CAD build for the part. Positions are in the model's coordinates, mm. Face numbers are marked on the shaded views. A direction names the side the tool comes from. Round coordinates to 2 decimals unless told otherwise and drop trailing zeros. Order: outer loops, then holes, each group sorted by start corner. A loop starts at its lowest first (then second) coordinate and runs counter-clockwise, first axis right, second up. Notation, with made-up numbers: (78.25, 19.5) - (108.25, 19.5) arc R8 cw to (108.25, 24.5) - close; hole circle Ø1 at (40, 73). An arc over 180 degrees is marked (long way). Write item = value, one per line.
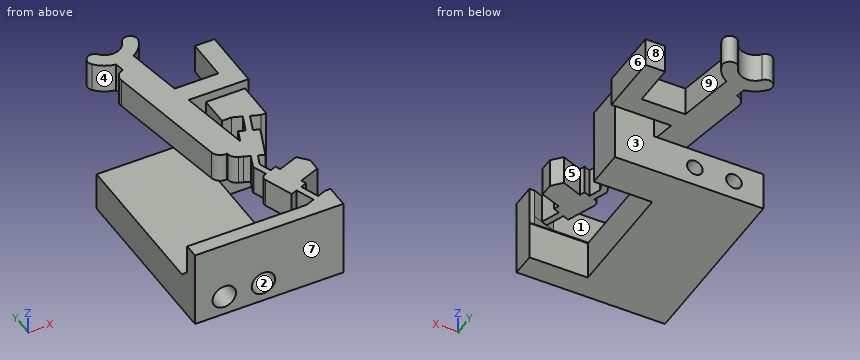
from build123d import *

# Parameters (mm, degrees)
BOSS_SWITCH_BODY_DEPTH            = 3
SKETCH1_W                         = 2.994375291
SKETCH1_H                         = 2.409101515
SKETCH1_W_2                       = 3.994375291
SKETCH1_H_2                       = 3.957767538
BOSS_FLANGE_WIDTH_DEPTH           = 5
BOSS_FLANGE_HEIGHT_REACH          = 36.354
SKETCH2_W                         = 4
SKETCH2_H                         = 3.957767538
SKETCH2_W_2                       = 8
SKETCH2_H_2                       = 1.451333978
SKETCH17_W                        = 15.1675
SKETCH17_H                        = 4
BOSS_FLANGE_SUPPORT_DEPTH         = 13.053634428
CUT_WALL_GAP_DEPTH                = 1
TAP_DRILL_FOR_M2X0_4_TAP1_D       = 1.6
M2_CLEARANCE_HOLE2_D              = 2.4
M2_CLEARANCE_HOLE2_DEPTH          = 13.462735941
CHAMFER_FLANGE_SUPPORT_3_SIZE     = 1
FILLET1_R                         = 1
FILLET2_R                         = 0.5
SKETCH28_W                        = 5.9675
SKETCH28_H                        = 12.095866891
CUT_PRINT_SUPPORT_CLEARANCE_DEPTH = 33.624103931


with BuildPart() as part:
    # Sketch-SwitchBossUp → Boss-Switch Body (new body)
    with BuildSketch(Plane.XY):
        with BuildLine():
            Line((-5.697895702, 26.949658376), (-5.524247524, 25.964850623))
            ThreePointArc((-5.524247524, 25.964850623), (-6.169751391, 25.553619307), (-6.3354071, 24.806394693))
            Line((-6.3354071, 24.806394693), (-4.07798079, 12.003893904))
            ThreePointArc((-4.07798079, 12.003893904), (-3.666749473, 11.358390037), (-2.919524859, 11.192734328))
            Line((-2.919524859, 11.192734328), (-2.795819507, 10.49116641))
            Line((-2.795819507, 10.49116641), (-1.8481327, 10.123820116))
            Line((-1.8481327, 10.123820116), (-1.21876104, 9.87986046))
            Line((-1.21876104, 9.87986046), (-1.735258621, 8.547390389))
            ThreePointArc((-1.735258621, 8.547390389), (-1.752158006, 8.457034961), (-1.735258621, 8.366679532))
            Line((-1.735258621, 8.366679532), (-1.21876104, 7.034209461))
            Line((-1.21876104, 7.034209461), (-1.8481327, 6.790249805))
            Line((-1.8481327, 6.790249805), (-0.547014535, 3.433600952))
            Line((-0.547014535, 3.433600952), (0.082357125, 3.677560608))
            Line((0.082357125, 3.677560608), (0.805200549, 1.81275569))
            Line((0.805200549, 1.81275569), (-0.12720191, 1.451333978))
            Line((-0.12720191, 1.451333978), (-0.12720191, 0))
            Line((-0.12720191, 0), (2.867173381, 0))
            Line((2.867173381, 0), (2.867173381, 2.409101515))
            Line((2.867173381, 2.409101515), (2.343664607, 2.409101515))
            Line((2.343664607, 2.409101515), (1.411262148, 2.047679803))
            Line((1.411262148, 2.047679803), (0.688418723, 3.912484721))
            Line((0.688418723, 3.912484721), (1.317790383, 4.156444377))
            Line((1.317790383, 4.156444377), (1.117265944, 4.673761056))
            Line((1.117265944, 4.673761056), (3.17940291, 5.473095148))
            Line((3.17940291, 5.473095148), (3.17940291, 6.808547192))
            Line((3.17940291, 6.808547192), (2.279218661, 7.795066081))
            Line((2.279218661, 7.795066081), (0.217196658, 6.995776551))
            Line((0.217196658, 6.995776551), (0.016672219, 7.51309323))
            Line((0.016672219, 7.51309323), (-0.612699441, 7.269133574))
            Line((-0.612699441, 7.269133574), (-1.038134762, 8.366679532))
            ThreePointArc((-1.038134762, 8.366679532), (-1.055034148, 8.457034961), (-1.038134762, 8.547390389))
            Line((-1.038134762, 8.547390389), (-0.612699441, 9.644936347))
            Line((-0.612699441, 9.644936347), (0.016672219, 9.400976691))
            Line((0.016672219, 9.400976691), (1.317790383, 12.757625544))
            Line((1.317790383, 12.757625544), (0.688418723, 13.0015852))
            Line((0.688418723, 13.0015852), (1.411262148, 14.866390118))
            Line((1.411262148, 14.866390118), (2.343664607, 14.504968406))
            Line((2.343664607, 14.504968406), (2.867173381, 14.504968406))
            Line((2.867173381, 14.504968406), (2.867173381, 18.462735944))
            Line((2.867173381, 18.462735944), (-0.111637615, 18.462735944))
            Line((-0.111637615, 18.462735944), (-1.12720191, 18.462735944))
            Line((-1.12720191, 18.462735944), (-1.12720191, 15.462735944))
            Line((-1.12720191, 15.462735944), (-0.12720191, 15.462735944))
            Line((-0.12720191, 15.462735944), (0.805200549, 15.101314231))
            Line((0.805200549, 15.101314231), (0.082357125, 13.236509313))
            Line((0.082357125, 13.236509313), (-0.547014535, 13.480468969))
            Line((-0.547014535, 13.480468969), (-1.059112089, 12.159350171))
            Line((-1.059112089, 12.159350171), (-2.346896051, 19.462735944))
            Line((-2.346896051, 19.462735944), (3.767173381, 19.462735944))
            Line((3.767173381, 19.462735944), (3.767173381, 25.857619356))
            Line((3.767173381, 25.857619356), (1.767173381, 25.857619356))
            Line((1.767173381, 25.857619356), (1.767173381, 21.462735944))
            Line((1.767173381, 21.462735944), (-2.699550012, 21.462735944))
            Line((-2.699550012, 21.462735944), (-3.728280196, 27.296954732))
            ThreePointArc((-3.728280196, 27.296954732), (-2.874356585, 27.992742953), (-2.319025652, 28.944012807))
            ThreePointArc((-2.319025652, 28.944012807), (-2.76728001, 29.905297381), (-3.728564583, 29.457043022))
            ThreePointArc((-3.728564583, 29.457043022), (-4.944660137, 28.436617692), (-6.436422172, 28.97957467))
            ThreePointArc((-6.436422172, 28.97957467), (-7.493046212, 29.072017295), (-7.585488837, 28.015393255))
            ThreePointArc((-7.585488837, 28.015393255), (-6.738295005, 27.311426358), (-5.697895702, 26.949658376))
        make_face()
    extrude(amount=BOSS_SWITCH_BODY_DEPTH)

    # Sketch1 → Boss-Flange Width (add)
    with BuildSketch(Plane(origin=(0, 0, 0), x_dir=(-1, 0, 0), z_dir=(0, 0, -1))):
        with Locations((-1.369985736, 1.204550758)):
            Rectangle(SKETCH1_W, SKETCH1_H)
        with Locations((-0.869985736, 16.483852175)):
            Rectangle(SKETCH1_W_2, SKETCH1_H_2)
    extrude(amount=BOSS_FLANGE_WIDTH_DEPTH)

    # Boss-Flange Height: up to this face of the body (flat: up to its plane)
    boss_flange_height_end = Plane(part.part.faces().sort_by_distance((-0.12720191, 1.077409098, -1.438016547))[0])
    # Sketch2 → Boss-Flange Height (add, up to the picked face)
    with BuildSketch(Plane(origin=(-12.300326619, 0, 0), x_dir=(0, 0, -1), z_dir=(1, 0, 0)), mode=Mode.PRIVATE) as boss_flange_height_sk1:
        with Locations((3, 16.483852175)):
            Rectangle(SKETCH2_W, SKETCH2_H)
    boss_flange_height_tool1 = split(extrude(boss_flange_height_sk1.sketch, amount=BOSS_FLANGE_HEIGHT_REACH, mode=Mode.PRIVATE), bisect_by=boss_flange_height_end, keep=Keep.BOTH, mode=Mode.PRIVATE)
    # Sketch2 → Boss-Flange Height (add, up to the picked face)
    with BuildSketch(Plane(origin=(-12.300326619, 0, 0), x_dir=(0, 0, -1), z_dir=(1, 0, 0)), mode=Mode.PRIVATE) as boss_flange_height_sk2:
        with Locations((1, 0.725666989)):
            Rectangle(SKETCH2_W_2, SKETCH2_H_2)
    boss_flange_height_tool2 = split(extrude(boss_flange_height_sk2.sketch, amount=BOSS_FLANGE_HEIGHT_REACH, mode=Mode.PRIVATE), bisect_by=boss_flange_height_end, keep=Keep.BOTH, mode=Mode.PRIVATE)
    add(boss_flange_height_tool1.solids().sort_by(Axis((-12.300327, 16.483852, -3), (1, 0, 0)))[0])
    add(boss_flange_height_tool2.solids().sort_by(Axis((-12.300327, 0.725667, -1), (1, 0, 0)))[0])

    # Sketch17 → Boss-Flange Support (add)
    with BuildSketch(Plane.XZ.offset(-1.451333978)):
        with Locations((-4.716576619, -3)):
            Rectangle(SKETCH17_W, SKETCH17_H)
    extrude(amount=-BOSS_FLANGE_SUPPORT_DEPTH)

    # Sketch27 → Cut-Wall Gap (cut)
    with BuildSketch(Plane.XY):
        Polygon((-0.12720191, 15.462735944), (2.343664607, 14.504968406), (-1.12720191, 14.504968406), (-1.12720191, 15.462735944), align=None)
        Polygon((2.343664607, 2.409101515), (-0.12720191, 2.409101515), (-0.12720191, 1.451333978), align=None)
    extrude(amount=-CUT_WALL_GAP_DEPTH, mode=Mode.SUBTRACT)

    # Tap Drill for M2x0.4 Tap1 (through all)
    with Locations(Plane(origin=(0, 0, 0), x_dir=(-1, 0, 0), z_dir=(0, -1, 0))):
        with Locations((9.300326619, 3), (5.300326619, 3)):
            Hole(TAP_DRILL_FOR_M2X0_4_TAP1_D / 2)

    # M2 Clearance Hole2
    with Locations(Plane.XZ):
        with Locations((-9.300326619, -3), (-5.300326619, -3)):
            Hole(M2_CLEARANCE_HOLE2_D / 2, depth=M2_CLEARANCE_HOLE2_DEPTH)

    # Chamfer-Flange Support 3
    chamfer_flange_support_3_edges = [part.edges().sort_by_distance(p)[0] for p in [
        (-6.213764264, 1.451333978, -1),
    ]]
    chamfer(chamfer_flange_support_3_edges, length=CHAMFER_FLANGE_SUPPORT_3_SIZE)

    # Fillet1
    fillet1_edges = [part.edges().sort_by_distance(p)[0] for p in [
        (-2.795819507, 10.49116641, 1.5),
    ]]
    fillet(fillet1_edges, radius=FILLET1_R)

    # Fillet2
    fillet2_edges = [part.edges().sort_by_distance(p)[0] for p in [
        (-1.8481327, 6.790249805, 1.5),
    ]]
    fillet(fillet2_edges, radius=FILLET2_R)

    # Sketch28 → Cut-Print Support Clearance (cut, through all)
    with BuildSketch(Plane.XY.offset(-1)):
        with Locations((-0.116576619, 8.457034961)):
            Rectangle(SKETCH28_W, SKETCH28_H)
    extrude(amount=-CUT_PRINT_SUPPORT_CLEARANCE_DEPTH, mode=Mode.SUBTRACT)


solid = part.part
(1) Drop flat-ended pins along their axis: pin 1 (1.5 mm diameter, centred on y = 6, z = 2, fed in from +X); pin 2 (3 mm diameter, centred on y = 12.5, z = 0, fed in from +X); pin 3 (1.5 mm diameter, centred on y = 23, z = 2, fed in from -X). Give the stop position or say it passes through.
Solved:
pin_1 = 3.18
pin_2 = 1.32
pin_3 = -6.15
(2) Band-saw the part on D-D on z = -1.5. List the corners of the cut face in (x, y).
Solved:
outline = (-12.3, 0) - (2.87, 0) - (2.87, 2.41) - (-3.1, 2.41) - (-3.1, 14.5) - (2.87, 14.5) - (2.87, 18.46) - (-12.3, 18.46) - close
(3) Band-saw the part on B-B on x = -9. List the corners of the cut face in (y, z).
Solved:
outline = (0, -5) - (18.46, -5) - (18.46, -3.74) - (13.46, -3.74) - (13.46, -4.16) - (0, -4.16) - close; (0, -1.84) - (13.46, -1.84) - (13.46, -2.26) - (18.46, -2.26) - (18.46, -1) - (2.45, -1) - (1.45, 0) - (1.45, 3) - (0, 3) - close
(4) Tool access for the marked faces 1, 2, 3, 4 and 5: list every direction of +Z, -Z, +X, -X, +Y, -Y with a clear straight run to the whole face (end or side of a thin tool).
Solved:
face_1 = +Z, -X
face_2 = -Y
face_3 = -Z, +X
face_4 = +Z, -Z, -X
face_5 = +Z, -Z
(5) Pull direction Y, two halves, no side cores. Call the marked faces 6, 7, 8 and 9: released by +Y, released by -Y, zero draft, split by the parting line, or undercut.
Solved:
face_6 = zero draft
face_7 = released by -Y
face_8 = released by +Y
face_9 = undercut
(6) Band-saw the part on C-C on y = 24. List the corners of the cut face in (x, z).
Solved:
outline = (-6.19, 0) - (-3.15, 0) - (-3.15, 3) - (-6.19, 3) - close; (1.77, 0) - (3.77, 0) - (3.77, 3) - (1.77, 3) - close
(7) Probe line 1 along X through (y, z) = (15.5, -3); line 2 along Y through (x, z) = (2.5, 2.75); line 3 along Y through (x, z) = (-2.25, -2.5). List the from-to ranges inside material, lowest first.
Solved:
line_1 = -12.3 to -10.1, -8.5 to -6.1, -4.5 to 2.87
line_2 = 0 to 2.41, 5.21 to 7.55, 14.5 to 18.46, 19.46 to 25.86
line_3 = 0 to 2.41, 14.5 to 18.46
(8) Band-saw the part on A-A on z = -3. List the corners of the cut face in (x, y).
Solved:
outline = (-12.3, 0) - (-10.5, 0) - (-10.5, 13.46) - (-10.1, 13.46) - (-10.1, 18.46) - (-12.3, 18.46) - close; (-8.5, 13.46) - (-8.1, 13.46) - (-8.1, 0) - (-6.5, 0) - (-6.5, 13.46) - (-6.1, 13.46) - (-6.1, 18.46) - (-8.5, 18.46) - close; (-4.5, 13.46) - (-4.1, 13.46) - (-4.1, 0) - (2.87, 0) - (2.87, 2.41) - (-3.1, 2.41) - (-3.1, 14.5) - (2.87, 14.5) - (2.87, 18.46) - (-4.5, 18.46) - close
